```python
from build123d import *

# Parameters (mm, degrees)
F0_W     = 100
F0_H     = 40
F1_DEPTH = 1
F2_W     = 95.8
F2_H     = 35.8
F2_W_2   = 93.8
F2_H_2   = 33.8
F3_DEPTH = 2
F4_R     = 1


with BuildPart() as f1:
    # F0 (on Top) → F1 (new body)
    with BuildSketch(Plane.XY):
        with Locations((50, 20)):
            Rectangle(F0_W, F0_H)
    extrude(amount=F1_DEPTH)

    # F2 (on face) → F3 (join)
    with BuildSketch(Plane.XY.offset(1)):
        with Locations((50, 20)):
            Rectangle(F2_W, F2_H)
        with Locations((50, 20)):
            Rectangle(F2_W_2, F2_H_2, mode=Mode.SUBTRACT)
    extrude(amount=F3_DEPTH)

    # F4
    f4_edges = [f1.edges().sort_by_distance(p)[0] for p in [
        (0, 0, 0.5),
        (100, 0, 0.5),
        (100, 40, 0.5),
        (0, 40, 0.5),
    ]]
    fillet(f4_edges, radius=F4_R)


solid = f1.part
```
Geometry: final body of the model. Coordinates: model frame, mm. A direction names the side the tool comes from. Coordinates: 2 decimals unless noted, no trailing zeros. Order: outer loops, then holes, each group sorted by start corner. A loop starts at its lowest first (then second) coordinate and runs counter-clockwise, first axis right, second up. Notation, with made-up numbers: M 74,-20.75 L 119,-20.75 A26 ccw 119,0.25 Z; hole C -1.5,17.25 d4. An arc over 180 degrees is marked long. Answer in a Markdown table with one row per item. Add a question column.
Q1. Contact query for flat-ended pins moving along their axis: P1, Ø1, axis at x = 61.5, z = 2, coming from the +Y side; P2, Ø12, axis at x = 36, y = 16.5, coming from the +Z side; P3, Ø1, axis at y = 32, z = 2.5, coming from the -X side. Output: stop coordinate, or through.
Q2. Section query A-A on z = 1.55. Return the cut outline in (x, y).
Q3. Line query: L1, parallel to Y at x = 15, z = 1.85; L2, parallel to X at y = 20, z = 1.1; L3, parallel to Z at x = 32, y = 14.5. Output: solid intervals per line, ascending.
Q4. Reachability of faces 1 (the flat face through (49, 2.1, 2)), 2 (the flat face through (49, 3.1, 2)), 3 (the flat face through (49, 37.9, 2)) from +Z, -Z, +X, -X, +Y, -Y: full face, straight path, thin tool, end or side. Return the list, or none.
Q5. Section query B-B on y = 6.5. Return the cut outline in (x, z).
Q6. Section query C-C on x = 76.5. Return the cut outline in (y, z).
Q7. Mould query, pull axis X, two halves, no side actions, for faces 4 (the flat face through (49, 36.9, 2)), 5 (the flat face through (97.9, 20, 2)), 6 (the flat face through (2.1, 20, 2)), 7 (the flat face through (49, 20, 0)). Classes: released by +X, released by -X, zero draft, split by the parting line, or undercut.
Completed:
| question | item | result |
|---|---|---|
| 1 | P1 | stops at y = 37.9 |
| 1 | P2 | stops at z = 1 |
| 1 | P3 | stops at x = 2.1 |
| 2 | outline | M 2.1,2.1 L 97.9,2.1 L 97.9,37.9 L 2.1,37.9 Z; hole M 3.1,3.1 L 96.9,3.1 L 96.9,36.9 L 3.1,36.9 Z |
| 3 | L1 | y = 2.1 to 3.1, 36.9 to 37.9 |
| 3 | L2 | x = 2.1 to 3.1, 96.9 to 97.9 |
| 3 | L3 | z = 0 to 1 |
| 4 | face 1 | +Z, +X, -X, -Y |
| 4 | face 2 | +Z |
| 4 | face 3 | +Z, +X, -X, +Y |
| 5 | outline | M 0,0 L 100,0 L 100,1 L 97.9,1 L 97.9,3 L 96.9,3 L 96.9,1 L 3.1,1 L 3.1,3 L 2.1,3 L 2.1,1 L 0,1 Z |
| 6 | outline | M 0,0 L 40,0 L 40,1 L 37.9,1 L 37.9,3 L 36.9,3 L 36.9,1 L 3.1,1 L 3.1,3 L 2.1,3 L 2.1,1 L 0,1 Z |
| 7 | face 4 | undercut |
| 7 | face 5 | released by +X |
| 7 | face 6 | released by -X |
| 7 | face 7 | zero draft |
